Work out the finished part from the listing and answer in its coordinate system (mm). Face numbers are marked on the shaded views. A direction names the side the tool comes from. Round coordinates to 2 decimals unless told otherwise and drop trailing zeros. Write each loop counter-clockwise with the first axis right and the second up, starting at its lowest first coordinate (ties: lowest second). Pieces come first, ordered by that corner, then holes. Notation, with made-up numbers: (-31.75, 54) - (2.25, 54) arc R15 ccw to (2.25, 59) - close; hole circle Ø11 at (52, 20.5). An arc over 180 degrees is marked (long way). Answer as a JSON object with one key per item and string values.
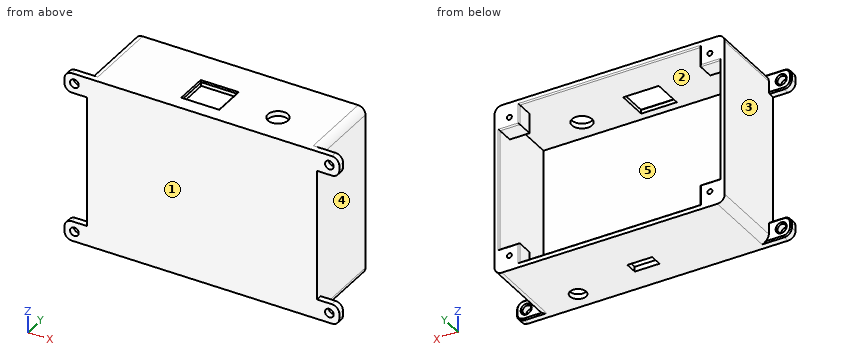
```python
from build123d import *

# Parameters (mm, degrees)
SKETCH1_R           = 1.75
BOSS_EXTRUDE1_DEPTH = 3
SKETCH2_W           = 92.99999868
SKETCH2_H           = 69.000001
SKETCH2_W_2         = 88.99999868
SKETCH2_H_2         = 65.000001
BOSS_EXTRUDE2_DEPTH = 30
SKETCH3_W           = 8
SKETCH3_H           = 8
SKETCH3_R           = 1
BOSS_EXTRUDE3_DEPTH = 15
CHAMFER1_SIZE       = 8
SKETCH4_R           = 3.25
CUT_EXTRUDE1_DEPTH  = 2
SKETCH5_W           = 14.3952
SKETCH5_H           = 12.269740894
CUT_EXTRUDE2_DEPTH  = 2
CHAMFER2_SIZE       = 0.5
FILLET1_R           = 3
CHAMFER4_SIZE       = 0.5
FILLET2_R           = 0.5
SKETCH6_R           = 4.05
CUT_EXTRUDE3_DEPTH  = 2
SKETCH7_W           = 10
SKETCH7_H           = 5
CUT_EXTRUDE4_DEPTH  = 2


with BuildPart() as part:
    # Sketch1 → Boss-Extrude1 (new body)
    with BuildSketch(Plane(origin=(0, 28.706829644, 0), x_dir=(-1, 0, 0), z_dir=(0, -1, 0))):
        with BuildLine():
            Line((27.769470492, -88.753133266), (-65.230528188, -88.753133266))
            Line((-65.230528188, -88.753133266), (-71.230528188, -88.753133266))
            ThreePointArc((-71.230528188, -88.753133266), (-73.351848531, -87.874453609), (-74.230528188, -85.753133266))
            Line((-74.230528188, -85.753133266), (-74.230528188, -83.753133266))
            ThreePointArc((-74.230528188, -83.753133266), (-73.351848531, -81.631812922), (-71.230528188, -80.753133266))
            Line((-71.230528188, -80.753133266), (-65.230528188, -80.753133266))
            Line((-65.230528188, -80.753133266), (-65.230528188, -27.753132266))
            Line((-65.230528188, -27.753132266), (-71.230528188, -27.753132266))
            ThreePointArc((-71.230528188, -27.753132266), (-73.351848531, -26.874452609), (-74.230528188, -24.753132266))
            Line((-74.230528188, -24.753132266), (-74.230528188, -22.753132266))
            ThreePointArc((-74.230528188, -22.753132266), (-73.351848531, -20.631811922), (-71.230528188, -19.753132266))
            Line((-71.230528188, -19.753132266), (-65.230528188, -19.753132266))
            Line((-65.230528188, -19.753132266), (27.769470492, -19.753132266))
            Line((27.769470492, -19.753132266), (33.769470492, -19.753132266))
            ThreePointArc((33.769470492, -19.753132266), (35.890790836, -20.631811922), (36.769470492, -22.753132266))
            Line((36.769470492, -22.753132266), (36.769470492, -24.753132266))
            ThreePointArc((36.769470492, -24.753132266), (35.890790836, -26.874452609), (33.769470492, -27.753132266))
            Line((33.769470492, -27.753132266), (27.769470492, -27.753132266))
            Line((27.769470492, -27.753132266), (27.769470492, -80.753133266))
            Line((27.769470492, -80.753133266), (33.769470492, -80.753133266))
            ThreePointArc((33.769470492, -80.753133266), (35.890790836, -81.631812922), (36.769470492, -83.753133266))
            Line((36.769470492, -83.753133266), (36.769470492, -85.753133266))
            ThreePointArc((36.769470492, -85.753133266), (35.890790836, -87.874453609), (33.769470492, -88.753133266))
            Line((33.769470492, -88.753133266), (27.769470492, -88.753133266))
        make_face()
        with Locations(Location((32.769470492, -23.753132266, 0), (0, 0, 180))):
            Circle(SKETCH1_R, mode=Mode.SUBTRACT)
        with Locations((-70.230528188, -23.753132266)):
            Circle(SKETCH1_R, mode=Mode.SUBTRACT)
        with Locations(Location((-70.230528188, -84.753133266, 0), (0, 0, 180))):
            Circle(SKETCH1_R, mode=Mode.SUBTRACT)
        with Locations((32.769470492, -84.753133266)):
            Circle(SKETCH1_R, mode=Mode.SUBTRACT)
    extrude(amount=BOSS_EXTRUDE1_DEPTH)

    # Sketch2 → Boss-Extrude2 (add)
    with BuildSketch(Plane(origin=(0, 28.706829644, 0), x_dir=(1, 0, 0), z_dir=(0, 1, 0))):
        with Locations((18.730528848, -54.253132766)):
            Rectangle(SKETCH2_W, SKETCH2_H)
        with Locations((18.730528848, -54.253132766)):
            Rectangle(SKETCH2_W_2, SKETCH2_H_2, mode=Mode.SUBTRACT)
    extrude(amount=BOSS_EXTRUDE2_DEPTH)

    # Sketch3 → Boss-Extrude3 (add)
    # profile 1 of 4: a face of its own
    with BuildSketch(Plane(origin=(0, 58.706829644, 0), x_dir=(1, 0, 0), z_dir=(0, 1, 0))):
        with Locations((-21.769470492, -25.753132266)):
            Rectangle(SKETCH3_W, SKETCH3_H)
        with Locations(Location((-21.769470492, -25.753132266, 0), (0, 0, 180))):
            Circle(SKETCH3_R, mode=Mode.SUBTRACT)
    # profile 2 of 4: a face of its own
    with BuildSketch(Plane(origin=(0, 58.706829644, 0), x_dir=(1, 0, 0), z_dir=(0, 1, 0))):
        with Locations((59.230528188, -25.753132266)):
            Rectangle(SKETCH3_W, SKETCH3_H)
        with Locations((59.230528188, -25.753132266)):
            Circle(SKETCH3_R, mode=Mode.SUBTRACT)
    # profile 3 of 4: a face of its own
    with BuildSketch(Plane(origin=(0, 58.706829644, 0), x_dir=(1, 0, 0), z_dir=(0, 1, 0))):
        with Locations((59.230528188, -82.753133266)):
            Rectangle(SKETCH3_W, SKETCH3_H)
        with Locations(Location((59.230528188, -82.753133266, 0), (0, 0, 180))):
            Circle(SKETCH3_R, mode=Mode.SUBTRACT)
    # profile 4 of 4: a face of its own
    with BuildSketch(Plane(origin=(0, 58.706829644, 0), x_dir=(1, 0, 0), z_dir=(0, 1, 0))):
        with Locations((-21.769470492, -82.753133266)):
            Rectangle(SKETCH3_W, SKETCH3_H)
        with Locations((-21.769470492, -82.753133266)):
            Circle(SKETCH3_R, mode=Mode.SUBTRACT)
    extrude(amount=-BOSS_EXTRUDE3_DEPTH)

    # Chamfer1
    # the kernel refuses this chamfer: 8 mm, written as the material it takes off along each edge
    with BuildSketch(Plane(origin=(-17.769470492, 43.706829644, 21.753132266), x_dir=(-0.9996219169112963, -0.027495876610600302, 0), z_dir=(0, 0, 1)), Plane(origin=(2.803993411, 43.706829644, 29.753132266), x_dir=(0, -0.027495876610596853, -0.9996219169112965), z_dir=(-1, 0, 0)), Plane(origin=(2.803993411, 43.706829644, 78.753133266), x_dir=(-1.3984416378867394e-14, 0.9996219169112965, -0.027495876610597703), z_dir=(-1, 0, 0)), Plane(origin=(-17.769470492, 43.706829644, 86.753133266), x_dir=(0.02749587661057268, 0.9996219169112972, -1.045466831585503e-14), z_dir=(0, 0, -1)), Plane(origin=(34.657064284, 43.706829644, 29.753132266), x_dir=(-1.4167575710639342e-14, 0.999621916911297, 0.0274958766105757), z_dir=(1, 0, 0)), Plane(origin=(55.230528188, 43.706829644, 21.753132266), x_dir=(-0.027495876610600312, 0.9996219169112963, -1.0650038269745103e-14), z_dir=(0, 0, 1))) as chamfer1_piece_1:
        Polygon((CHAMFER1_SIZE * 0.999621916911, -CHAMFER1_SIZE * 0.0274958766106), (-CHAMFER1_SIZE * 0.0274958766106, -CHAMFER1_SIZE * 0.999621916911), (0, 0), align=None)
    extrude(amount=28.573463904, mode=Mode.SUBTRACT)
    with BuildSketch(Plane(origin=(55.230528188, 43.706829644, 86.753133266), x_dir=(-0.027495876610600312, 0.9996219169112963, -1.0259298361964941e-14), z_dir=(0, 0, -1)), Plane(origin=(34.657064284, 43.706829644, 78.753133266), x_dir=(-1.4082101355812438e-14, 0.9996219169112965, -0.027495876610597703), z_dir=(1, 0, 0))) as chamfer1_piece_2:
        Polygon((CHAMFER1_SIZE * 0.999621916911, CHAMFER1_SIZE * 0.0274958766106), (-CHAMFER1_SIZE * 0.0274958766106, CHAMFER1_SIZE * 0.999621916911), (0, 0), align=None)
    extrude(amount=28.573463904, mode=Mode.SUBTRACT)

    # Sketch4 → Cut-Extrude1 (cut)
    with BuildSketch(Plane(origin=(0, 0, 19.753132266), x_dir=(-1, 0, 0), z_dir=(0, 0, -1))):
        with Locations(Location((-46.555528188, 33.301829644, 0), (0, 0, 90))):
            Circle(SKETCH4_R)
    extrude(amount=-CUT_EXTRUDE1_DEPTH, mode=Mode.SUBTRACT)

    # Sketch5 → Cut-Extrude2 (cut)
    with BuildSketch(Plane.XY.offset(88.753133266)):
        with Locations((14.645530209, 38.12231703)):
            Rectangle(SKETCH5_W, SKETCH5_H)
    extrude(amount=-CUT_EXTRUDE2_DEPTH, mode=Mode.SUBTRACT)

    # Chamfer2
    chamfer2_edges = [part.edges().sort_by_distance(p)[0] for p in [
        (7.447930209, 38.12231703, 88.753133266),
        (14.645530209, 31.987446583, 88.753133266),
        (21.843130209, 38.12231703, 88.753133266),
        (14.645530209, 44.257187477, 88.753133266),
    ]]
    chamfer(chamfer2_edges, length=CHAMFER2_SIZE)

    # Fillet1
    fillet1_edges = [part.edges().sort_by_distance(p)[0] for p in [
        (-27.769470492, 43.706829644, 19.753132266),
        (-27.769470492, 43.706829644, 88.753133266),
        (65.230528188, 43.706829644, 88.753133266),
        (65.230528188, 43.706829644, 19.753132266),
    ]]
    fillet(fillet1_edges, radius=FILLET1_R)

    # Chamfer4
    chamfer4_edges = [part.edges().sort_by_distance(p)[0] for p in [
        (66.730528188, 28.706829644, 88.753133266),
        (73.351848531, 28.706829644, 87.874453609),
        (74.230528188, 28.706829644, 84.753133266),
        (73.351848531, 28.706829644, 81.631812922),
        (68.230528188, 28.706829644, 80.753133266),
        (68.230528188, 28.706829644, 27.753132266),
        (73.351848531, 28.706829644, 26.874452609),
        (74.230528188, 28.706829644, 23.753132266),
        (73.351848531, 28.706829644, 20.631811922),
        (-29.269470492, 28.706829644, 19.753132266),
        (-35.890790836, 28.706829644, 20.631811922),
        (-36.769470492, 28.706829644, 23.753132266),
        (-35.890790836, 28.706829644, 26.874452609),
        (-30.769470492, 28.706829644, 27.753132266),
        (-30.769470492, 28.706829644, 80.753133266),
        (-35.890790836, 28.706829644, 81.631812922),
        (-36.769470492, 28.706829644, 84.753133266),
        (-35.890790836, 28.706829644, 87.874453609),
        (-34.519470492, 28.706829644, 23.753132266),
        (71.980528188, 28.706829644, 23.753132266),
        (68.480528188, 28.706829644, 84.753133266),
        (-31.019470492, 28.706829644, 84.753133266),
        (-29.269470492, 28.706829644, 88.753133266),
        (66.730528188, 28.706829644, 19.753132266),
    ]]
    chamfer(chamfer4_edges, length=CHAMFER4_SIZE)

    # Fillet2
    fillet2_edges = [part.edges().sort_by_distance(p)[0] for p in [
        (-25.769470492, 58.706829644, 54.253132766),
        (-21.769470492, 58.706829644, 29.753132266),
        (-17.769470492, 58.706829644, 25.753132266),
        (18.730528848, 58.706829644, 21.753132266),
        (55.230528188, 58.706829644, 25.753132266),
        (59.230528188, 58.706829644, 29.753132266),
        (63.230528188, 58.706829644, 54.253132766),
        (59.230528188, 58.706829644, 78.753133266),
        (55.230528188, 58.706829644, 82.753133266),
        (18.730528848, 58.706829644, 86.753133266),
        (-17.769470492, 58.706829644, 82.753133266),
        (-21.769470492, 58.706829644, 78.753133266),
    ]]
    fillet(fillet2_edges, radius=FILLET2_R)

    # Sketch6 → Cut-Extrude3 (cut)
    with BuildSketch(Plane.XY.offset(88.753133266)):
        with Locations((42.343130209, 37.706829644)):
            Circle(SKETCH6_R)
    extrude(amount=-CUT_EXTRUDE3_DEPTH, mode=Mode.SUBTRACT)

    # Sketch7 → Cut-Extrude4 (cut)
    with BuildSketch(Plane(origin=(0, 0, 19.753132266), x_dir=(-1, 0, 0), z_dir=(0, 0, -1))):
        with Locations((-17.230528188, 38.206829644)):
            Rectangle(SKETCH7_W, SKETCH7_H)
    extrude(amount=-CUT_EXTRUDE4_DEPTH, mode=Mode.SUBTRACT)


solid = part.part
```
Item 1: A cutting plane is placed at A-A (x = 16). Write down the section's boundary in (y, z), and give its area (3 significant figures).
Results found:
{"outline": "(25.71, 19.75) - (35.71, 19.75) - (35.71, 21.75) - (28.71, 21.75) - (28.71, 86.75) - (31.99, 86.75) - (31.99, 88.25) - (31.49, 88.75) - (25.71, 88.75) - close; (40.71, 19.75) - (58.71, 19.75) - (58.71, 21.25) arc R0.5 ccw to (58.21, 21.75) - (40.71, 21.75) - close; (44.26, 86.75) - (58.21, 86.75) arc R0.5 ccw to (58.71, 87.25) - (58.71, 88.75) - (44.76, 88.75) - (44.26, 88.25) - close", "area": "292 mm²"}
Item 2: Consider line 1 along Z through (x, y) = (60.5, 39); line 2 along X through (y, z) = (47, 63.5); line 3 along Z through (x, y) = (55.5, 52.5). Determine where each line is inside the solid, lowest interval first.
Results found:
{"line 1": "19.75 to 21.75, 86.75 to 88.75", "line 2": "-27.77 to -25.77, 63.23 to 65.23", "line 3": "19.75 to 29.75, 78.75 to 88.75"}
Item 3: A cutting plane is placed at C-C (x = 27.5). Write down the section's boundary in (y, z).
Results found:
{"outline": "(25.71, 19.75) - (58.71, 19.75) - (58.71, 21.25) arc R0.5 ccw to (58.21, 21.75) - (28.71, 21.75) - (28.71, 86.75) - (58.21, 86.75) arc R0.5 ccw to (58.71, 87.25) - (58.71, 88.75) - (25.71, 88.75) - close"}
Item 4: For the marked faces 1 and 2, determine the directions among +Z, -Z, +X, -X, +Y, -Y from which every point of the face is accessible in a straight line to the end or side of a thin tool.
Results found:
{"face 1": "+Z, -Z, +X, -X, -Y", "face 2": "none"}
Item 5: A cutting plane is placed at B-B (z = 36). Write down the section's boundary in (x, y).
Results found:
{"outline": "(-27.77, 25.71) - (65.23, 25.71) - (65.23, 58.71) - (63.73, 58.71) arc R0.5 ccw to (63.23, 58.21) - (63.23, 28.71) - (-25.77, 28.71) - (-25.77, 58.21) arc R0.5 ccw to (-26.27, 58.71) - (-27.77, 58.71) - close"}
Item 6: Determine the mould class of the marked faces 3, 4 and 5 for opening direction X: pulls with the +X half, pulls with the -X half, needs draft (parallel to the pull), parting line crosses it, or undercut.
Results found:
{"face 3": "pulls with the -X half", "face 4": "pulls with the +X half", "face 5": "undercut"}
Item 7: Each of these flat-tipped pins is pushed along its axis until it touches: P1, Ø1.6, axis at y = 35.5, z = 88, coming from the +X side; P2, Ø2, axis at y = 53.5, z = 81.5, coming from the +X side; P3, Ø1.8, axis at x = 59.23, z = 25.75, coming from the +Y side. Where does it stop, or does it pass through?
Results found:
{"P1": "x = 64.86", "P2": "x = 65.23", "P3": "y = 28.71"}
